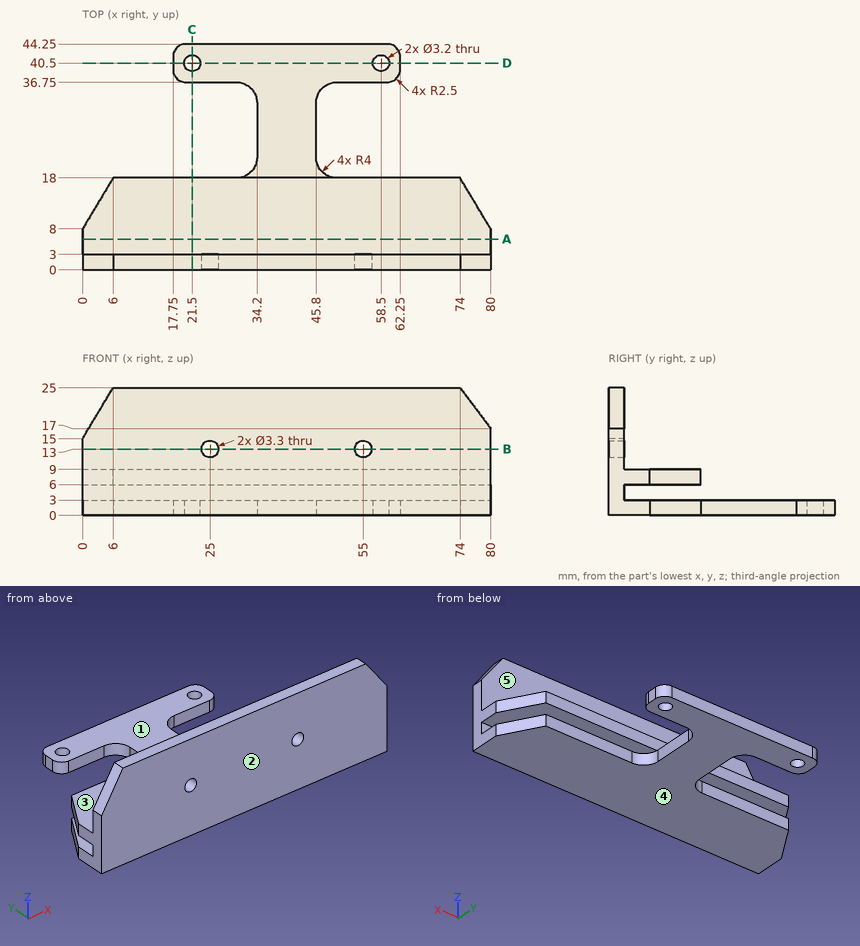
Could you check a few things on this drawing? It's one solid part, dimensions in mm from its lowest x, y, z. A direction names the side the tool comes from. Give positions to 0.01 mm unless a question says otherwise; leave off trailing zeros. Write each loop counter-clockwise with the first axis right and the second up, starting at its lowest first coordinate (ties: lowest second). Pieces come first, ordered by that corner, then holes. Notation, with made-up numbers: (30.5, -25) -> (45.5, -25) arc R24 ccw to (45.5, -2) -> close; hole circle Ø3 at (25.25, 71.25). An arc over 180 degrees is marked (long way). Answer as a JSON object with one key per item and string values.
Q1. Suppose I cut it at D-D on y = 40.5. Write out the boundary of the cut face in (x, z).
Taken from the geometry:
{"outline": "(17.75, 0) -> (19.9, 0) -> (19.9, 3) -> (17.75, 3) -> close; (23.1, 0) -> (56.9, 0) -> (56.9, 3) -> (23.1, 3) -> close; (60.1, 0) -> (62.25, 0) -> (62.25, 3) -> (60.1, 3) -> close"}
Q2. We'd pull the mould along Z, two halves only. Please class the marked faces 1, 2 and 3: released by +Z, released by -Z, zero draft, split by the parting line, or undercut.
Taken from the geometry:
{"face 1": "undercut", "face 2": "zero draft", "face 3": "released by +Z"}
Q3. Suppose I cut it at C-C on x = 21.5. Write out the boundary of the cut face in (y, z), then the cut area to 3 significant figures.
Taken from the geometry:
{"outline": "(0, 0) -> (18, 0) -> (18, 3) -> (3, 3) -> (3, 6) -> (18, 6) -> (18, 9) -> (3, 9) -> (3, 25) -> (0, 25) -> close; (36.75, 0) -> (38.9, 0) -> (38.9, 3) -> (36.75, 3) -> close; (42.1, 0) -> (44.25, 0) -> (44.25, 3) -> (42.1, 3) -> close", "area": "178 mm²"}
Q4. Which directions (+Z, -Z, +X, -X, +Y, -Y) give clear straight access to the entire face, cutting with the end or side of a thin tool? Please do the marked faces 4 and 5.
Taken from the geometry:
{"face 4": "-Z, +X, -X, +Y, -Y", "face 5": "+Z, +X, -X, +Y"}
Q5. Please list where these lines run through material, in increasing order: L1, parallel to Y at x = 58.5, z = 1.2; L2, parallel to X at y = 0.85, z = 13; L3, parallel to Z at x = 41, y = 9.
Taken from the geometry:
{"L1": "y = 0 to 18, 36.75 to 38.9, 42.1 to 44.25", "L2": "x = 0 to 23.35, 26.65 to 53.35, 56.65 to 80", "L3": "z = 0 to 3, 6 to 9"}
Q6. Suppose I cut it at A-A on y = 6. Write out the boundary of the cut face in (x, z).
Taken from the geometry:
{"outline": "(0, 0) -> (80, 0) -> (80, 3) -> (0, 3) -> close; (0, 6) -> (80, 6) -> (80, 9) -> (0, 9) -> close"}
Q7. Will these pins go through, and if not, where does the flat tip stop? pin 1 Ø20.5 at (x, y) = (28, 30.5) entering from +Z; pin 2 Ø1.5 at (x, z) = (30, 7) entering from +Y; pin 3 Ø1.5 at (x, z) = (53.5, 4) entering from +Y; pin 4 Ø8 at (y, z) = (7.5, 18.5) entering from -X.
Taken from the geometry:
{"pin 1": "stops at z = 3", "pin 2": "stops at y = 18", "pin 3": "stops at y = 3", "pin 4": "passes through"}
Q8. Suppose I cut it at B-B on z = 13. Write out the boundary of the cut face in (x, y), then the cut area to 3 significant figures.
Taken from the geometry:
{"outline": "(0, 0) -> (23.35, 0) -> (23.35, 3) -> (0, 3) -> close; (26.65, 0) -> (53.35, 0) -> (53.35, 3) -> (26.65, 3) -> close; (56.65, 0) -> (80, 0) -> (80, 3) -> (56.65, 3) -> close", "area": "220 mm²"}
